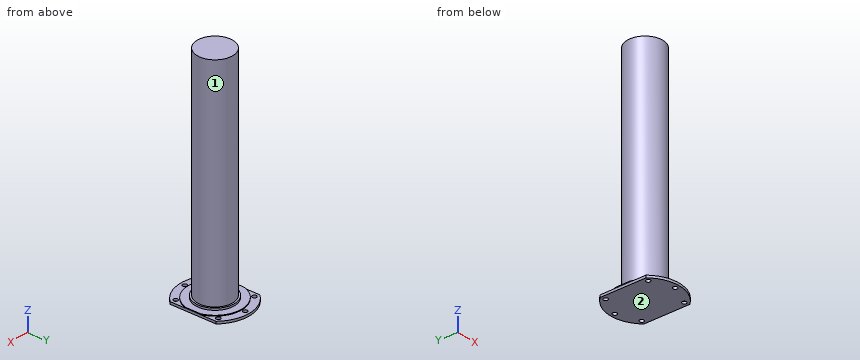
```python
from build123d import *

# Parameters (mm, degrees)
F0_R     = 5.0292
F1_DEPTH = 5.5118
F2_R     = 45.3771
F3_DEPTH = 6.35
F5_DEPTH = 1.778
F6_R     = 41.5036
F7_DEPTH = 508


with BuildPart() as f1:
    # F0 (on Top) → F1 (new body)
    with BuildSketch(Plane.XY):
        with BuildLine():
            Line((61.47253, -51.707207), (58.887924, 54.632588))
            ThreePointArc((58.887924, 54.632588), (-1.951797, 80.303784), (-61.47253, 51.707207))
            Line((-61.47253, 51.707207), (-58.887924, -54.632588))
            ThreePointArc((-58.887924, -54.632588), (1.951797, -80.303784), (61.47253, -51.707207))
        make_face()
        with Locations((-48.229271, -50.632113)):
            Circle(F0_R, mode=Mode.SUBTRACT)
        with Locations((1.699066, -69.905555)):
            Circle(F0_R, mode=Mode.SUBTRACT)
        with Locations((50.632113, -48.229271)):
            Circle(F0_R, mode=Mode.SUBTRACT)
        with Locations((-50.632113, 48.229271)):
            Circle(F0_R, mode=Mode.SUBTRACT)
        with Locations((-1.699066, 69.905555)):
            Circle(F0_R, mode=Mode.SUBTRACT)
        with Locations((48.229271, 50.632113)):
            Circle(F0_R, mode=Mode.SUBTRACT)
    extrude(amount=F1_DEPTH)

    # F2 (on face) → F3 (join)
    with BuildSketch(Plane.XY.offset(5.5118)):
        Circle(F2_R)
    extrude(amount=F3_DEPTH)

    # F4 (on face) → F5 (join)
    with BuildSketch(Plane.XY.offset(5.5118)):
        with BuildLine():
            Line((-60.592857, 15.514361), (-59.767597, -18.439742))
            ThreePointArc((-59.767597, -18.439742), (1.519779, -62.529033), (60.592857, -15.514361))
            Line((60.592857, -15.514361), (59.767597, 18.439742))
            ThreePointArc((59.767597, 18.439742), (-1.519779, 62.529033), (-60.592857, 15.514361))
        make_face()
    extrude(amount=F5_DEPTH)

    # F6 (on face) → F7 (join)
    with BuildSketch(Plane.XY.offset(11.8618)):
        Circle(F6_R)
    extrude(amount=F7_DEPTH)


solid = f1.part
```
Model file for the job. Use its own axes, mm. Face numbers are marked on the shaded views. A direction names the side the tool comes from. Coordinates: 2 decimals unless noted, no trailing zeros. Write each loop counter-clockwise with the first axis right and the second up, starting at its lowest first coordinate (ties: lowest second). Pieces come first, ordered by that corner, then holes. Notation, with made-up numbers: (-2, 23.25) - (39, 23.25) arc R25 cw to (39, 60.25) - close; hole circle Ø2 at (77.5, 54.5). An arc over 180 degrees is marked (long way). Use a Markdown table: item, result. Add a question column.
Item 1: Drop flat-ended pins along their axis: pin 1 (2 mm diameter, centred on x = -19, z = 229.5, fed in from +Y); pin 2 (3 mm diameter, centred on y = 4, z = 352, fed in from +X); pin 3 (3 mm diameter, centred on x = -30, z = 94, fed in from -Y); pin 4 (9 mm diameter, centred on x = 1.7, y = -69.91, fed in from +Z). Give the stop position or say it passes through.
Item 2: Band-saw the part on A-A, the plane y = 32. Write the cut outline in (x, z).
Item 3: Band-saw the part on C-C, the plane z = 123.5. Write the cut outline in (x, y), and give its area (3 significant figures).
Item 4: Band-saw the part on D-D, the plane y = -4.5. Write the cut outline in (x, z), and give its area (3 significant figures).
Item 5: Drill centre lines: line 1 along Z through (x, y) = (50, 7); line 2 along Z through (x, y) = (-17.5, 64.5); line 3 along X through (y, z) = (1.5, 444). Where is each one in solid material? Low to high.
Item 6: Band-saw the part on B-B, the plane x = 28.5. Write the cut outline in (y, z).
Item 7: 3-axis set-ups, long thin cutter, end or side, ignore diameter. For the marked faces 1 and 2: which of +Z, -Z, +X, -X, +Y, -Y reach the whole face in a straight line?
A:
| question | item | result |
|---|---|---|
| 1 | pin 1 | stops at y = 37.4 |
| 1 | pin 2 | stops at x = 41.43 |
| 1 | pin 3 | stops at y = -30.17 |
| 1 | pin 4 | passes through |
| 2 | outline | (-60.99, 0) - (59.44, 0) - (59.44, 5.51) - (53.74, 5.51) - (53.74, 7.29) - (32.17, 7.29) - (32.17, 11.86) - (26.43, 11.86) - (26.43, 519.86) - (-26.43, 519.86) - (-26.43, 11.86) - (-32.17, 11.86) - (-32.17, 7.29) - (-53.74, 7.29) - (-53.74, 5.51) - (-60.99, 5.51) - close |
| 3 | outline | circle Ø83.01 at (0, 0) |
| 3 | area | 5,410 mm² |
| 4 | outline | (-60.11, 0) - (60.33, 0) - (60.33, 7.29) - (45.15, 7.29) - (45.15, 11.86) - (41.26, 11.86) - (41.26, 519.86) - (-41.26, 519.86) - (-41.26, 11.86) - (-45.15, 11.86) - (-45.15, 7.29) - (-60.11, 7.29) - close |
| 4 | area | 43,200 mm² |
| 5 | line 1 | z = 0 to 7.29 |
| 5 | line 2 | z = 0 to 5.51 |
| 5 | line 3 | x = -41.48 to 41.48 |
| 6 | outline | (-75.1, 0) - (75.1, 0) - (75.1, 5.51) - (55.68, 5.51) - (55.68, 7.29) - (35.31, 7.29) - (35.31, 11.86) - (30.17, 11.86) - (30.17, 519.86) - (-30.17, 519.86) - (-30.17, 11.86) - (-35.31, 11.86) - (-35.31, 7.29) - (-55.68, 7.29) - (-55.68, 5.51) - (-75.1, 5.51) - close |
| 7 | face 1 | +Z |
| 7 | face 2 | -Z, +X, -X, +Y, -Y |
